Geometry check sheet. Reference: drawing and pictorial views, mm from the part's lowest x, y, z. A direction names the side the tool comes from. Round coordinates to 2 decimals unless told otherwise and drop trailing zeros. Order: outer loops, then holes, each group sorted by start corner. A loop starts at its lowest first (then second) coordinate and runs counter-clockwise, first axis right, second up.
Q1. Scan lines: probe 1 along Z at (x, y) = (0.9, 14); probe 2 along X at (y, z) = (3.75, 11.5). Record each from-to range of solid material in increasing order.
Q2. Depth check by flat-ended pin: P1, Ø1, axis at y = 13.5, z = 6, coming from the -X side; P2, Ø0.9, axis at x = 0.5, y = 8.5, coming from the -Z side. Enter the tip coordinate at first touch or a pass-through.
Q3. Cross-section at B-B on x = 1.05. Record the cut outline in (y, z).
Q4. Cross-section at A-A on y = 7.75. Record the cut outline in (x, z).
Q5. Set-up check for the marked faces 1 and 2: record each of +Z, -Z, +X, -X, +Y, -Y from which the full face is reachable in a straight line by a thin tool's end or side.
Q6. Cross-section at C-C on z = 7.5. Record the cut outline in (x, y), then the cut area to 3 significant figures.
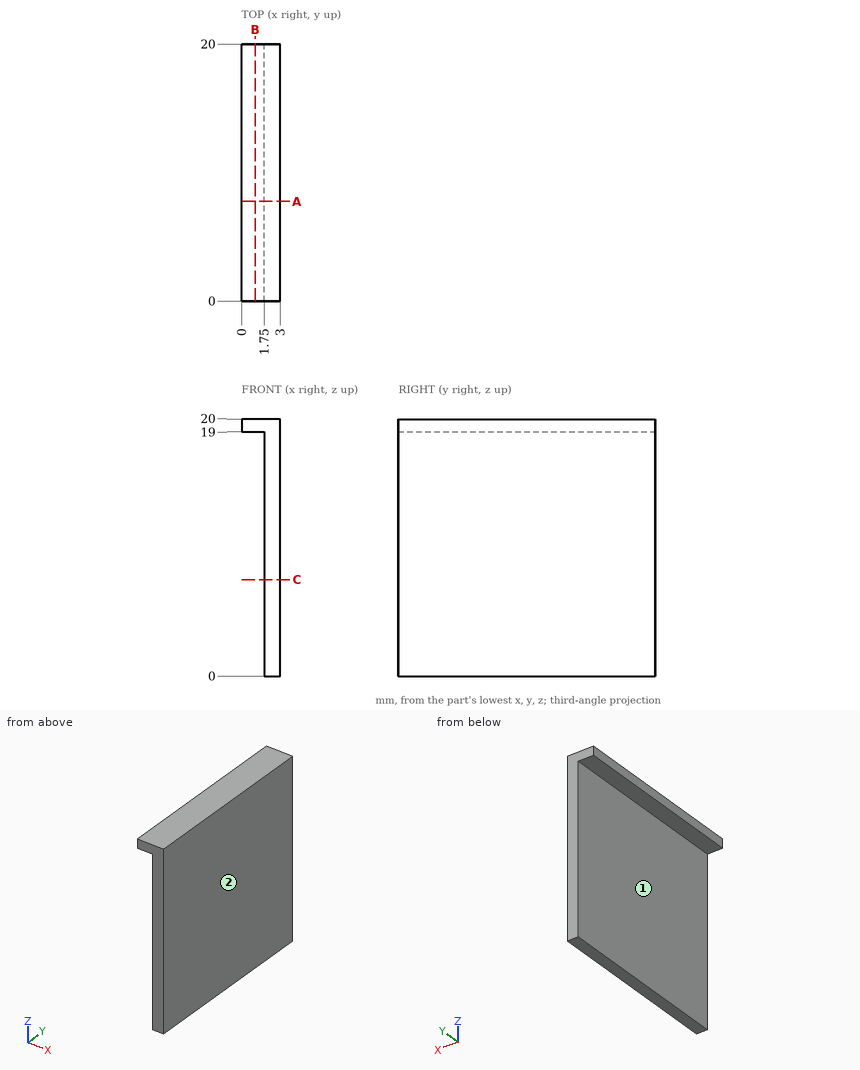
Results found:
1. probe 1: z = 19 to 20
1. probe 2: x = 1.75 to 3
2. P1: stops at x = 1.75
2. P2: stops at z = 19
3. outline: (0, 19) - (20, 19) - (20, 20) - (0, 20) - close
4. outline: (0, 19) - (1.75, 19) - (1.75, 0) - (3, 0) - (3, 20) - (0, 20) - close
5. face 1: -Z, -X, +Y, -Y
5. face 2: +Z, -Z, +X, +Y, -Y
6. outline: (1.75, 0) - (3, 0) - (3, 20) - (1.75, 20) - close
6. area: 25.0 mm2
